For this review, use the dimensioned drawing (mm, ordinates from the lowest corner) and the shaded views. A direction names the side the tool comes from. Round coordinates to 2 decimals unless told otherwise and drop trailing zeros. Write each loop counter-clockwise with the first axis right and the second up, starting at its lowest first coordinate (ties: lowest second). Pieces come first, ordered by that corner, then holes. Notation, with made-up numbers: M 37.5,-30 L 74.5,-30 A25 ccw 74.5,5 Z; hole C -9,-39 d2. An arc over 180 degrees is marked long. Use one line per item in the form item = value. Start each with the question number.
Item 1: For P1, Ø10, axis at x = 45.5, y = 26, coming from the -Z side (1 decimal); P2, Ø23, axis at x = 37.5, z = 27, coming from the +Y side; P3, Ø3, axis at y = 19.5, z = 25.5, coming from the -X side, all flat-tipped, find the tip position at first contact; note any pin that passes through.
Item 2: For line 1 (Y direction, x = 27, z = 22); line 2 (X direction, y = 13, z = 64.5); line 3 (X direction, y = 38, z = 72) (1 decimal), list the stretches that pass through material, from the lowest coordinate up. Write a range as [from, to].
Item 3: Draft analysis for pull direction X (two halves, no side actions). For the marked faces 3, 4 and 5, state which applies: released by +X, released by -X, zero draft, split by the parting line, or undercut.
Item 4: For the marked faces 1 and 2, list the 3-axis set-ups (+Z, -Z, +X, -X, +Y, -Y) from which the entire face can be reached by the end or side of a thin tool; tool diameter is ignored.
Item 5: Add section A-A (y = 38). State the section outline as (x, z) points.
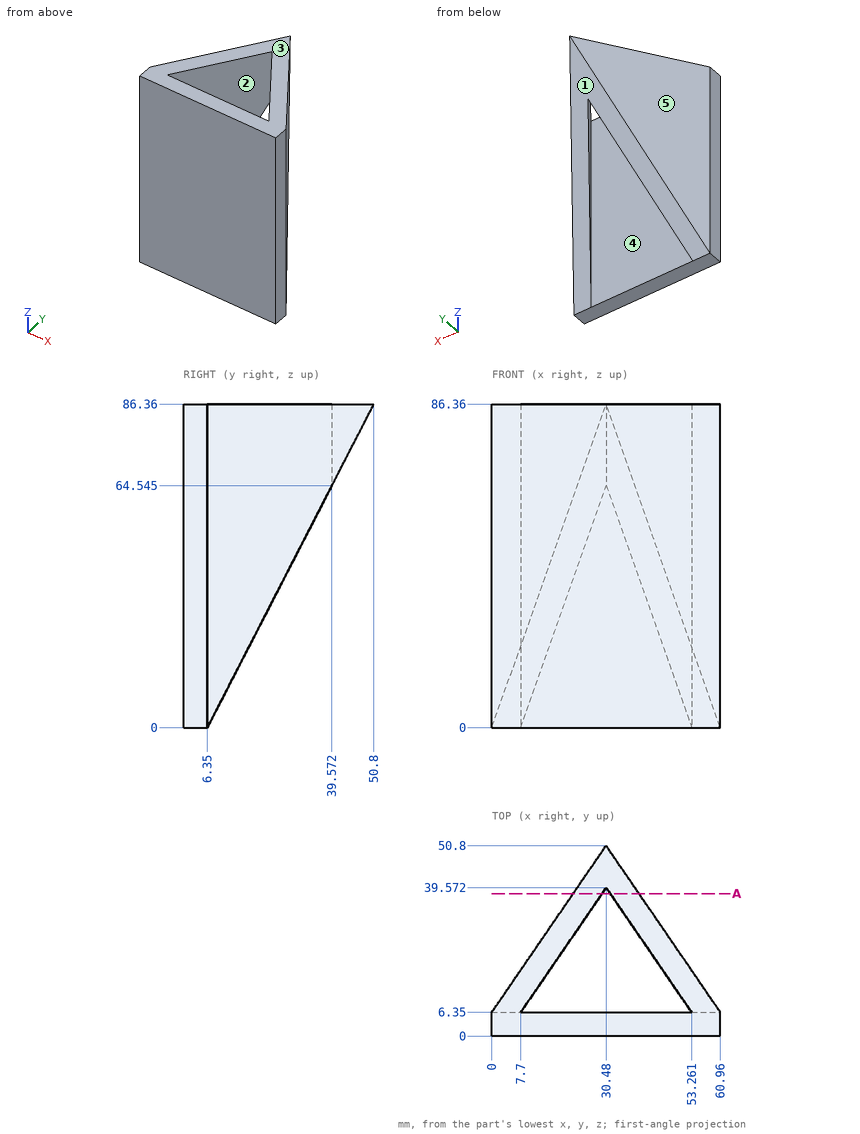
Calculated:
q1.P1 = 28.5
q1.P2 = 26.05
q1.P3 = 7.99
q2.line_1 = [0, 6.35]
q2.line_2 = [4.56, 12.26], [48.7, 56.4]
q2.line_3 = [21.7, 29.4], [31.6, 39.3]
q3.face_3 = zero draft
q3.face_4 = undercut
q3.face_5 = released by -X
q4.face_1 = -Z, +X, -X, +Y
q4.face_2 = +Z, -Z
q5.outline = M 21.7,61.49 L 29.4,61.49 L 29.4,86.36 L 21.7,86.36 Z; M 31.56,61.49 L 39.26,61.49 L 39.26,86.36 L 31.56,86.36 Z
